CAD build for the part. Positions are in the model's coordinates, mm. Face numbers are marked on the shaded views. A direction names the side the tool comes from. Coordinates: 2 decimals unless noted, no trailing zeros. Order: outer loops, then holes, each group sorted by start corner. A loop starts at its lowest first (then second) coordinate and runs counter-clockwise, first axis right, second up. Notation, with made-up numbers: (-27.75, 26.25) - (24.25, 26.25) arc R20 ccw to (24.25, 57.25) - close; hole circle Ø1 at (-22, 13.5). An arc over 180 degrees is marked (long way). Use one line per item in the form item = value.
```python
from build123d import *

# Parameters (mm, degrees)
F1_DEPTH = 50.8
F3_D     = 6.35
F4_R     = 5.08


with BuildPart() as f1:
    # F0 (on Front) → F1 (new body)
    with BuildSketch(Plane.XZ):
        Polygon((6.35, 6.35), (6.35, 25.4), (0, 25.4), (0, 0), (50.8, 0), (50.8, 25.4), (44.45, 25.4), (44.45, 6.35), align=None)
    extrude(amount=F1_DEPTH)

    # F3 (through all)
    with Locations(Plane(origin=(0, 0, 0), x_dir=(0, -1, 0), z_dir=(-1, 0, 0))):
        with Locations((25.4, 12.7)):
            Hole(F3_D / 2)

    # F4
    f4_edges = [f1.edges().sort_by_distance(p)[0] for p in [
        (50.8, -25.4, 25.4),
        (47.625, -50.8, 25.4),
        (47.625, 0, 25.4),
    ]]
    fillet(f4_edges, radius=F4_R)


solid = f1.part
```
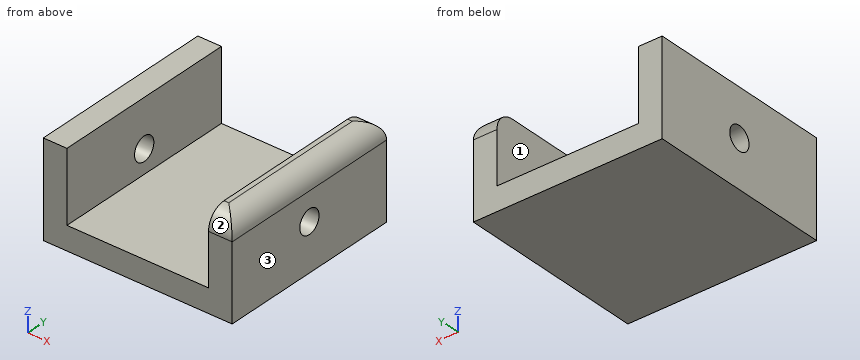
Item 1: 3-axis set-ups, long thin cutter, end or side, ignore diameter. For the marked faces 1, 2 and 3: which of +Z, -Z, +X, -X, +Y, -Y reach the whole face in a straight line?
Derived:
face_1 = +Z, +Y, -Y
face_2 = +Z, +X, -Y
face_3 = +Z, -Z, +X, +Y, -Y
Item 2: Cut at B-B, the plane y = -25.4. Write the cut outline in (x, z) (3 decimals), plus the area to 3 significant figures.
Derived:
outline = (0, 0) - (50.8, 0) - (50.8, 9.525) - (44.45, 9.525) - (44.45, 6.35) - (6.35, 6.35) - (6.35, 9.525) - (0, 9.525) - close; (0, 15.875) - (6.35, 15.875) - (6.35, 25.4) - (0, 25.4) - close; (44.45, 15.875) - (50.8, 15.875) - (50.8, 20.32) arc R5.08 ccw to (45.72, 25.4) - (44.45, 25.4) - close
area = 478 mm²
Item 3: Cut at D-D, the plane y = -14. Write the cut outline in (x, z), plus the area to 3 significant figures.
Derived:
outline = (0, 0) - (50.8, 0) - (50.8, 20.32) arc R5.08 ccw to (45.72, 25.4) - (44.45, 25.4) - (44.45, 6.35) - (6.35, 6.35) - (6.35, 25.4) - (0, 25.4) - close
area = 559 mm²
Item 4: Cut at C-C, the plane z = 8.25. Write the cut outline in (x, y).
Derived:
outline = (0, -50.8) - (6.35, -50.8) - (6.35, 0) - (0, 0) - close; (44.45, -50.8) - (50.8, -50.8) - (50.8, 0) - (44.45, 0) - close
Item 5: Drop flat-ended pins along their axis: pin 1 (5.5 mm diameter, centred on y = -26, z = 17.5, fed in from -X); pin 2 (10 mm diameter, centred on x = 39, y = -41, fed in from +Z). Give the stop position or say it passes through.
Derived:
pin_1 = 0
pin_2 = 6.35
Item 6: Drill centre lines: line 1 (X direction, y = -11, z = 7.5); line 2 (Z direction, x = 5, y = -25.4) (3 decimals); line 3 (Z direction, x = 31.5, y = -23.5). Where is each one in solid material? Low to high. Write a range as [from, to].
Derived:
line_1 = [0, 6.35], [44.45, 50.8]
line_2 = [0, 9.525], [15.875, 25.4]
line_3 = [0, 6.35]
Item 7: Cut at A-A, the plane z = 12.7. Write the cut outline in (x, y) (3 decimals), plus the area to 3 significant figures.
Derived:
outline = (0, -50.8) - (6.35, -50.8) - (6.35, -28.575) - (0, -28.575) - close; (0, -22.225) - (6.35, -22.225) - (6.35, 0) - (0, 0) - close; (44.45, -50.8) - (50.8, -50.8) - (50.8, -28.575) - (44.45, -28.575) - close; (44.45, -22.225) - (50.8, -22.225) - (50.8, 0) - (44.45, 0) - close
area = 565 mm²
